Part model, mm, in its own coordinate system. Face numbers are marked on the shaded views. A direction names the side the tool comes from. Round coordinates to 2 decimals unless told otherwise and drop trailing zeros. Write each loop counter-clockwise with the first axis right and the second up, starting at its lowest first coordinate (ties: lowest second). Pieces come first, ordered by that corner, then holes.
```python
from build123d import *

# Parameters (mm, degrees)
SKETCH1_R           = 50
BOSS_EXTRUDE1_DEPTH = 20
SKETCH4_R           = 50
BOSS_EXTRUDE2_DEPTH = 40
BOSS_EXTRUDE2_TAPER = 9
SKETCH3_7_R         = 52
BOSS_EXTRUDE4_DEPTH = 2


with BuildPart() as part:
    # Sketch1 → Boss-Extrude1 (new body)
    with BuildSketch(Plane.XY):
        Circle(SKETCH1_R)
    extrude(amount=-BOSS_EXTRUDE1_DEPTH)

    # Sketch4 → Boss-Extrude2 (add)
    with BuildSketch(Plane(origin=(0, 0, -20), x_dir=(-1, 0, 0), z_dir=(0, 0, -1))):
        with Locations(Location((0, 0, 0), (0, 0, 180))):
            Circle(SKETCH4_R)
    extrude(amount=BOSS_EXTRUDE2_DEPTH, taper=BOSS_EXTRUDE2_TAPER)

    # Loft2: read off the stored shape, not the designer's step
    # Loft2: loft between two sections, ruled curve by curve
    loft2_from = [
        Edge.make_bspline([(-0.09152616, 45.31531343, 58.435490337), (1.991803683, 45.318769716, 58.437102029), (4.206873224, 45.205331996, 58.384205151), (8.88600843, 44.645276274, 58.123046879), (11.350748929, 44.198388733, 57.914659797), (16.473473932, 42.853465541, 57.287511813), (19.132143408, 41.954695988, 56.868408687), (24.523466482, 39.583734538, 55.762811206), (27.256405564, 38.110209758, 55.075695316), (32.597052055, 34.493832776, 53.389351035), (35.204002583, 32.349251741, 52.389316475), (38.814480974, 28.61367569, 50.647388755), (39.967462866, 27.282788702, 50.02678596), (42.134576019, 24.458220553, 48.709668201), (43.14861453, 22.964518438, 48.013143466), (45.000389489, 19.831572212, 46.552226648), (45.838021163, 18.192337872, 45.787839122), (47.303056553, 14.794522163, 44.203411636), (47.930358248, 13.035986558, 43.383393016), (48.947497256, 9.433887898, 41.703706825), (49.337252793, 7.590405028, 40.844076645), (49.861578346, 3.858952965, 39.104071973), (49.99610264, 1.971088931, 38.223746516), (50.00372982, -1.805187188, 36.462840042), (49.876832475, -3.693484925, 35.582312346), (49.367583678, -7.426651708, 33.841508086), (48.985277522, -9.271415445, 32.981280629), (47.982696048, -12.876864862, 31.300031954), (47.36250218, -14.637470087, 30.479048255), (45.911202122, -18.040124056, 28.892364651), (45.080197767, -19.682126696, 28.126686245), (43.241090789, -22.82119617, 26.66291411), (42.2330929, -24.318252884, 25.9648251), (40.077404144, -27.149992649, 24.644363161), (38.929806111, -28.484696346, 24.021980606), (35.334441818, -32.232227035, 22.274478346), (32.736171819, -34.385443637, 21.270416955), (27.410169514, -38.019516805, 19.575820807), (24.683201066, -39.502099682, 18.884481058), (19.301491648, -41.89093381, 17.770549409), (16.646470579, -42.798518884, 17.347335539), (11.529212738, -44.160430414, 16.712265763), (9.066293964, -44.615493042, 16.500066575), (4.389452468, -45.191070517, 16.23167039), (2.174856003, -45.311857144, 16.175346661), (-1.991803683, -45.318769716, 16.172123276), (-4.206873224, -45.205331996, 16.225020153), (-8.88600843, -44.645276274, 16.486178425), (-11.350748929, -44.198388733, 16.694565508), (-16.473473932, -42.853465541, 17.321713492), (-19.132143408, -41.954695988, 17.740816618), (-24.523466482, -39.583734538, 18.846414099), (-27.256405564, -38.110209758, 19.533529988), (-32.597052055, -34.493832776, 21.21987427), (-35.204002583, -32.349251741, 22.21990883), (-38.814480974, -28.61367569, 23.96183655), (-39.967462866, -27.282788702, 24.582439345), (-42.134576019, -24.458220553, 25.899557104), (-43.14861453, -22.964518438, 26.596081839), (-45.000389489, -19.831572212, 28.056998657), (-45.838021163, -18.192337872, 28.821386183), (-47.303056553, -14.794522163, 30.405813669), (-47.930358248, -13.035986558, 31.225832289), (-48.947497256, -9.433887898, 32.905518479), (-49.337252793, -7.590405028, 33.76514866), (-49.861578346, -3.858952965, 35.505153332), (-49.99610264, -1.971088931, 36.385478789), (-50.00372982, 1.805187188, 38.146385262), (-49.876832475, 3.693484925, 39.026912958), (-49.367583678, 7.426651708, 40.767717218), (-48.985277522, 9.271415445, 41.627944676), (-47.982696048, 12.876864862, 43.30919335), (-47.36250218, 14.637470087, 44.13017705), (-45.911202122, 18.040124056, 45.716860654), (-45.080197767, 19.682126696, 46.48253906), (-43.241090789, 22.82119617, 47.946311195), (-42.2330929, 24.318252884, 48.644400205), (-40.077404144, 27.149992649, 49.964862143), (-38.929806111, 28.484696346, 50.587244699), (-35.334441818, 32.232227035, 52.334746958), (-32.736171819, 34.385443637, 53.338808349), (-27.410169514, 38.019516805, 55.033404498), (-24.683201066, 39.502099682, 55.724744247), (-19.301491648, 41.89093381, 56.838675895), (-16.646470579, 42.798518884, 57.261889765), (-11.529212738, 44.160430414, 57.896959542), (-9.066293964, 44.615493042, 58.10915873), (-4.389452468, 45.191070517, 58.377554915), (-2.174856003, 45.311857144, 58.433878644), (-0.09152616, 45.31531343, 58.435490337)], [0, 0, 0, 0, 0.03125, 0.03125, 0.0625, 0.0625, 0.09375, 0.09375, 0.125, 0.125, 0.15625, 0.15625, 0.171875, 0.171875, 0.1875, 0.1875, 0.203125, 0.203125, 0.21875, 0.21875, 0.234375, 0.234375, 0.25, 0.25, 0.265625, 0.265625, 0.28125, 0.28125, 0.296875, 0.296875, 0.3125, 0.3125, 0.328125, 0.328125, 0.34375, 0.34375, 0.375, 0.375, 0.40625, 0.40625, 0.4375, 0.4375, 0.46875, 0.46875, 0.5, 0.5, 0.53125, 0.53125, 0.5625, 0.5625, 0.59375, 0.59375, 0.625, 0.625, 0.65625, 0.65625, 0.671875, 0.671875, 0.6875, 0.6875, 0.703125, 0.703125, 0.71875, 0.71875, 0.734375, 0.734375, 0.75, 0.75, 0.765625, 0.765625, 0.78125, 0.78125, 0.796875, 0.796875, 0.8125, 0.8125, 0.828125, 0.828125, 0.84375, 0.84375, 0.875, 0.875, 0.90625, 0.90625, 0.9375, 0.9375, 0.96875, 0.96875, 1, 1, 1, 1], 3),
    ]
    loft2_to = [
        Edge.make_bspline([(0.136420865, 44.999793214, 0), (2.011412249, 44.994109012, 0), (4.004403567, 44.871769265, 0), (8.21287139, 44.295142718, 0), (10.428953936, 43.840585304, 0), (15.032858325, 42.482621984, 0), (17.421293091, 41.578484294, 0), (22.261978921, 39.200460503, 0), (24.714480484, 37.725249561, 0), (29.503544757, 34.110714545, 0), (31.839417938, 31.969677001, 0), (35.070773805, 28.244344926, 0), (36.102019394, 26.917691058, 0), (38.03876047, 24.10333168, 0), (38.944172383, 22.615605767, 0), (40.595623515, 19.496398085, 0), (41.341568486, 17.864926477, 0), (42.643679265, 14.484388202, 0), (43.199753477, 12.735367429, 0), (44.097775949, 9.153930324, 0), (44.439650999, 7.321593977, 0), (44.893522054, 3.613861762, 0), (45.005477417, 1.738570519, 0), (44.994109012, -2.011412249, 0), (44.870785588, -3.885990223, 0), (44.394442444, -7.590902411, 0), (44.041463999, -9.421132248, 0), (43.121743345, -12.997058703, 0), (42.555074828, -14.742675783, 0), (41.232491368, -18.115257064, 0), (40.476668297, -19.742175929, 0), (38.806335385, -22.851313328, 0), (37.891919851, -24.333522272, 0), (35.93815057, -27.136087223, 0), (34.898880272, -28.456464139, 0), (31.644996659, -32.162135635, 0), (29.296185043, -34.288971141, 0), (24.485293431, -37.87440304, 0), (22.023892564, -39.33471705, 0), (17.168877462, -41.683347464, 0), (14.775004701, -42.572987164, 0), (10.162951439, -43.903011492, 0), (7.944153589, -44.344124173, 0), (3.732266966, -44.895223668, 0), (1.738570519, -45.005477417, 0), (-2.011412249, -44.994109012, 0), (-4.004403567, -44.871769265, 0), (-8.21287139, -44.295142718, 0), (-10.428953936, -43.840585304, 0), (-15.032858325, -42.482621984, 0), (-17.421293091, -41.578484294, 0), (-22.261978921, -39.200460503, 0), (-24.714480484, -37.725249561, 0), (-29.503544757, -34.110714545, 0), (-31.839417938, -31.969677001, 0), (-35.070773805, -28.244344926, 0), (-36.102019394, -26.917691058, 0), (-38.03876047, -24.10333168, 0), (-38.944172383, -22.615605767, 0), (-40.595623515, -19.496398085, 0), (-41.341568486, -17.864926477, 0), (-42.643679265, -14.484388202, 0), (-43.199753477, -12.735367429, 0), (-44.097775949, -9.153930324, 0), (-44.439650999, -7.321593977, 0), (-44.893522054, -3.613861762, 0), (-45.005477417, -1.738570519, 0), (-44.994109012, 2.011412249, 0), (-44.870785588, 3.885990223, 0), (-44.394442444, 7.590902411, 0), (-44.041463999, 9.421132248, 0), (-43.121743345, 12.997058703, 0), (-42.555074828, 14.742675783, 0), (-41.232491368, 18.115257064, 0), (-40.476668297, 19.742175929, 0), (-38.806335385, 22.851313328, 0), (-37.891919851, 24.333522272, 0), (-35.93815057, 27.136087223, 0), (-34.898880272, 28.456464139, 0), (-31.644996659, 32.162135635, 0), (-29.296185043, 34.288971141, 0), (-24.485293431, 37.87440304, 0), (-22.023892564, 39.33471705, 0), (-17.168877462, 41.683347464, 0), (-14.775004701, 42.572987164, 0), (-10.162951439, 43.903011492, 0), (-7.944153589, 44.344124173, 0), (-3.732266966, 44.895223668, 0), (-1.738570519, 45.005477417, 0), (0.136420865, 44.999793214, 0)], [0, 0, 0, 0, 0.03125, 0.03125, 0.0625, 0.0625, 0.09375, 0.09375, 0.125, 0.125, 0.15625, 0.15625, 0.171875, 0.171875, 0.1875, 0.1875, 0.203125, 0.203125, 0.21875, 0.21875, 0.234375, 0.234375, 0.25, 0.25, 0.265625, 0.265625, 0.28125, 0.28125, 0.296875, 0.296875, 0.3125, 0.3125, 0.328125, 0.328125, 0.34375, 0.34375, 0.375, 0.375, 0.40625, 0.40625, 0.4375, 0.4375, 0.46875, 0.46875, 0.5, 0.5, 0.53125, 0.53125, 0.5625, 0.5625, 0.59375, 0.59375, 0.625, 0.625, 0.65625, 0.65625, 0.671875, 0.671875, 0.6875, 0.6875, 0.703125, 0.703125, 0.71875, 0.71875, 0.734375, 0.734375, 0.75, 0.75, 0.765625, 0.765625, 0.78125, 0.78125, 0.796875, 0.796875, 0.8125, 0.8125, 0.828125, 0.828125, 0.84375, 0.84375, 0.875, 0.875, 0.90625, 0.90625, 0.9375, 0.9375, 0.96875, 0.96875, 1, 1, 1, 1], 3),
    ]
    loft2 = Solid(Shell([*[Face.make_surface_from_curves(loft2_from[k], loft2_to[k]) for k in range(1)], Face(Wire(loft2_from)), Face(Wire(loft2_to))]))
    add(loft2)

    # Sketch3<7> → Boss-Extrude4 (add)
    with BuildSketch(Plane(origin=(0, -14.288495613, 30.641777725), x_dir=(1, 0, 0), z_dir=(0, -0.4226182617407003, 0.9063077870366496))):
        with Locations(Location((0, 15.765610554, 0), (0, 0, 270))):
            Circle(SKETCH3_7_R)
    extrude(amount=-BOSS_EXTRUDE4_DEPTH)


solid = part.part
```
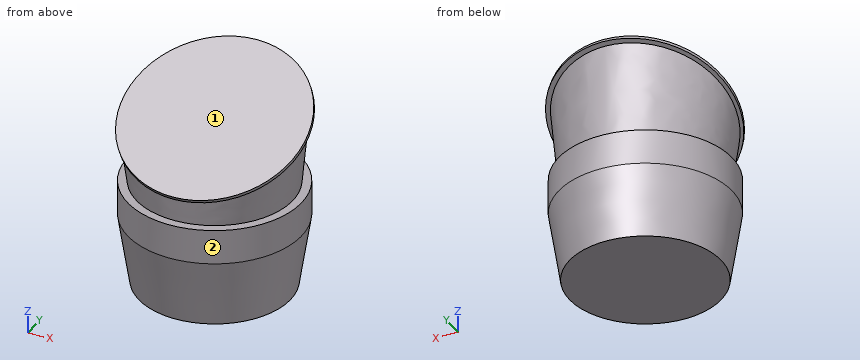
Q1. Which spindle directions (+Z, -Z, +X, -X, +Y, -Y) get a long thin tool onto all of the face, cutting with end or side? Do the marked faces 1 and 2. Say none if no direction does.
Values follow:
face 1: +Z, +X, -X, -Y
face 2: -Z
Q2. Drop flat-ended pins along their axis: pin 1 (10 mm diameter, centred on y = -11.5, z = 0, fed in from -X); pin 2 (1.5 mm diameter, centred on y = 28.5, z = 11, fed in from +X); pin 3 (5 mm diameter, centred on x = 34.5, z = -35, fed in from -Y). Give the stop position or say it passes through.
Values follow:
pin 1: stops at x = -49.58
pin 2: stops at x = 36.32
pin 3: stops at y = -35.33
Q3. Wall check: L1, parallel to X at y = 2, z = 14.5; L2, parallel to Z at x = 10, y = 6.5; L3, parallel to Y at x = -33.5, z = -47. Give the ranges that are in metal, low to high.
Values follow:
L1: x = -46.85 to 46.85
L2: z = -60 to 40.34
L3: y = -31.12 to 31.12
Q4. Cut at A-A on z = -43.5. Write the cut outline in (x, y), plus the area to 3 significant figures.
Values follow:
outline: circle Ø92.56 at (0, 0)
area: 6,730 mm2
